For this review, take the finished solid that the model builds, in its own axes (mm). A direction names the side the tool comes from. Round coordinates to 2 decimals unless told otherwise and drop trailing zeros. Write each loop counter-clockwise with the first axis right and the second up, starting at its lowest first coordinate (ties: lowest second). Pieces come first, ordered by that corner, then holes. Notation, with made-up numbers: (31, 56.25) -> (90, 56.25) arc R29 cw to (90, 91.25) -> close; hole circle Ø5 at (72.25, 41). An arc over 180 degrees is marked (long way). Answer as CSV lines item,"result". Start each with the question number.
Item 1: Take a section at C-C on y = 3. Give the boundary of the cut face in (x, z), then the cut area to 3 significant figures.
Item 2: For pin 1 Ø3 at (x, y) = (2, 13) entering from +Z; pin 2 Ø2 at (y, z) = (6, 0) entering from +X; pin 3 Ø6 at (x, y) = (-3.5, 2.5) entering from +Z, all flat-tipped, find the tip position at first contact; note any pin that passes through.
Item 3: Take a section at B-B on z = 0. Give the boundary of the cut face in (x, y), then the cut area to 3 significant figures.
Item 4: Wall thickness on probe 1 along Z at (x, y) = (0, 7); probe 2 along Z at (x, y) = (2.25, 7); probe 3 along Y at (x, z) = (-1.75, 2): over which ranges is each line inside the solid? List them lowest first. Write a range as from..to.
Item 5: Machinability: for faces 1 (the cylindrical face through (-1.08, 15.49, 4.88)), 2 (the cylindrical face through (-0.338, 6.803, -2.578)), which of the approach directions +Z, -Z, +X, -X, +Y, -Y give a long, thin tool a straight path to every point of the face, cutting with its end or side? Answer none if there is none.
Item 6: Take a section at A-A on x = 0. Give the boundary of the cut face in (y, z), then the cut area to 3 significant figures.
```python
from build123d import *

# Parameters (mm, degrees)
SKETCH1_R           = 2.6
BOSS_EXTRUDE1_DEPTH = 15
SKETCH2_R           = 5
BOSS_EXTRUDE2_DEPTH = 2
CHAMFER1_SIZE       = 1.2
CHAMFER2_SIZE       = 1


with BuildPart() as part:
    # Sketch1 → Boss-Extrude1 (new body)
    with BuildSketch(Plane(origin=(0, 0, 0), x_dir=(1, 0, 0), z_dir=(0, 1, 0))):
        Circle(SKETCH1_R)
    extrude(amount=BOSS_EXTRUDE1_DEPTH)

    # Sketch2 → Boss-Extrude2 (add)
    with BuildSketch(Plane(origin=(0, 15, 0), x_dir=(1, 0, 0), z_dir=(0, 1, 0))):
        Circle(SKETCH2_R)
    extrude(amount=BOSS_EXTRUDE2_DEPTH)

    # Chamfer1
    chamfer1_edges = [part.edges().sort_by_distance(p)[0] for p in [
        (-2.6, 15, 0),
    ]]
    chamfer(chamfer1_edges, length=CHAMFER1_SIZE)

    # Chamfer2
    chamfer2_edges = [part.edges().sort_by_distance(p)[0] for p in [
        (-5, 17, 0),
    ]]
    chamfer(chamfer2_edges, length=CHAMFER2_SIZE)


solid = part.part
```
Output values:
1,outline,"circle Ø5.2 at (0, 0)"
1,area,"21.2 mm^2"
2,pin 1,"stops at z = 2.85"
2,pin 2,"stops at x = 2.6"
2,pin 3,"stops at z = 2.55"
3,outline,"(-5, 15) -> (-3.8, 15) -> (-2.6, 13.8) -> (-2.6, 0) -> (2.6, 0) -> (2.6, 13.8) -> (3.8, 15) -> (5, 15) -> (5, 16) -> (4, 17) -> (-4, 17) -> (-5, 16) -> close"
3,area,"98.4 mm^2"
4,probe 1,"z = -2.6..2.6"
4,probe 2,"z = -1.3..1.3"
4,probe 3,"y = 13.86..17"
5,face 1,"+Y, -Y"
5,face 2,"-Y"
6,outline,"(0, -2.6) -> (13.8, -2.6) -> (15, -3.8) -> (15, -5) -> (16, -5) -> (17, -4) -> (17, 4) -> (16, 5) -> (15, 5) -> (15, 3.8) -> (13.8, 2.6) -> (0, 2.6) -> close"
6,area,"98.4 mm^2"
